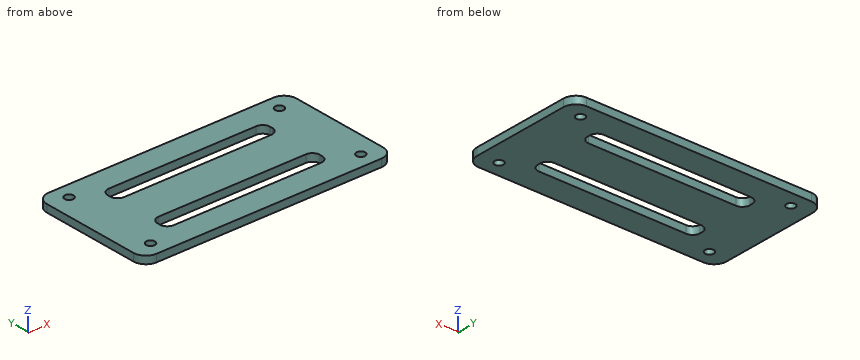
from build123d import *

# Parameters (mm, degrees)
F0_W     = 100
F0_H     = 50
F1_DEPTH = 3
F2_D     = 3.5
F2_DEPTH = 16
F3_R     = 5
F4_W     = 65
F4_H     = 7
F5_DEPTH = 25
F6_R     = 3


with BuildPart() as f1:
    # F0 (on Top) → F1 (new body)
    with BuildSketch(Plane.XY):
        Rectangle(F0_W, F0_H)
    extrude(amount=F1_DEPTH)

    # F2
    with Locations(Plane(origin=(0, 0, 0), x_dir=(1, 0, 0), z_dir=(0, 0, -1))):
        with Locations((-42.15, 18.85), (-42.15, -18.85), (42.15, 18.85), (42.15, -18.85)):
            Hole(F2_D / 2, depth=F2_DEPTH)

    # F3
    f3_edges = [f1.edges().sort_by_distance(p)[0] for p in [
        (-50, 25, 1.5),
        (-50, -25, 1.5),
        (50, 25, 1.5),
        (50, -25, 1.5),
    ]]
    fillet(f3_edges, radius=F3_R)

    # F4 (on face) → F5 (cut)
    with BuildSketch(Plane.XY.offset(3)):
        with Locations((0, 11.5)):
            Rectangle(F4_W, F4_H)
        with Locations((0, -11.5)):
            Rectangle(F4_W, F4_H)
    extrude(amount=-F5_DEPTH, mode=Mode.SUBTRACT)

    # F6
    f6_edges = [f1.edges().sort_by_distance(p)[0] for p in [
        (-32.5, 15, 1.5),
        (-32.5, 8, 1.5),
        (-32.5, -15, 1.5),
        (32.5, 8, 1.5),
        (32.5, -15, 1.5),
        (32.5, 15, 1.5),
        (32.5, -8, 1.5),
        (-32.5, -8, 1.5),
    ]]
    fillet(f6_edges, radius=F6_R)


solid = f1.part
Part model, mm, in its own coordinate system. Give positions to 0.01 mm unless a question says otherwise; leave off trailing zeros. Loops run counter-clockwise (first coordinate to the right, second up) from the corner with the lowest first, then second, coordinate; pieces in that order, holes last.
(1) Band-saw the part on B-B (x = 20). Write the cut outline in (y, z).
Return value:
outline: (-25, 0) - (-15, 0) - (-15, 3) - (-25, 3) - close; (-8, 0) - (8, 0) - (8, 3) - (-8, 3) - close; (15, 0) - (25, 0) - (25, 3) - (15, 3) - close
(2) Band-saw the part on C-C (z = 1.75). Write the cut outline in (x, y).
Return value:
outline: (-50, -20) arc R5 ccw to (-45, -25) - (45, -25) arc R5 ccw to (50, -20) - (50, 20) arc R5 ccw to (45, 25) - (-45, 25) arc R5 ccw to (-50, 20) - close; hole circle Ø3.5 at (-42.15, -18.85); hole circle Ø3.5 at (-42.15, 18.85); hole (-32.5, -12) arc R3 ccw to (-29.5, -15) - (29.5, -15) arc R3 ccw to (32.5, -12) - (32.5, -11) arc R3 ccw to (29.5, -8) - (-29.5, -8) arc R3 ccw to (-32.5, -11) - close; hole (-32.5, 11) arc R3 ccw to (-29.5, 8) - (29.5, 8) arc R3 ccw to (32.5, 11) - (32.5, 12) arc R3 ccw to (29.5, 15) - (-29.5, 15) arc R3 ccw to (-32.5, 12) - close; hole circle Ø3.5 at (42.15, -18.85); hole circle Ø3.5 at (42.15, 18.85)
(3) Drill centre lines: line 1 along Y through (x, z) = (-42.15, 2.35); line 2 along Y through (x, z) = (7.5, 1.9); line 3 along X through (y, z) = (-18.85, 1.9). Where is each one in solid material? Low to high.
Return value:
line 1: y = -25 to -20.6, -17.1 to 17.1, 20.6 to 25
line 2: y = -25 to -15, -8 to 8, 15 to 25
line 3: x = -50 to -43.9, -40.4 to 40.4, 43.9 to 50
(4) Pin check, flat tip, straight feed: pin 1 (1.5 mm diameter, centred on x = -12, y = -10.5, fed in from -Z). Stop position of the tip, or through.
Return value:
pin 1: passes through
(5) Band-saw the part on A-A (y = 18.85). Write the cut outline in (x, z), and give its area (3 significant figures).
Return value:
outline: (-50, 0) - (-43.9, 0) - (-43.9, 3) - (-50, 3) - close; (-40.4, 0) - (40.4, 0) - (40.4, 3) - (-40.4, 3) - close; (43.9, 0) - (50, 0) - (50, 3) - (43.9, 3) - close
area: 279 mm2
